Autodesk Inventor part; units mm, degrees
ref_plane "Work Plane1" through (0, 25, 0) normal (0, 1, 0) x (-1, 0, 0)
ref_plane "YZ Plane" through (0, 0, 0) normal (1, 0, 0) x (0, 1, 0)
ref_plane "XY Plane" through (0, 0, 0) normal (0, 0, 1) x (1, 0, 0)
sketch "Sketch1" plane through (0, 0, 0) normal (0, 1, 0) x (-1, 0, 0)
  line L0 (20, 50) -> (-20, 50)
  line L1 (-20, 50) -> (-20, -50)
  line L2 (-20, -50) -> (20, -50)
  line L3 (20, -50) -> (20, 50)
  line L4 (15, 45) -> (-15, 45)
  line L5 (-15, 45) -> (-15, -45)
  line L6 (-15, -45) -> (15, -45)
  line L7 (15, -45) -> (15, 45)
  line L8 (15, -45) -> (15, -50)
  line L9 (-15, -45) -> (-15, -50)
  point P0 (0, 0)
  dimension "d0" = 40
  dimension "d1" = 100
  dimension "d2" = 20
  dimension "d3" = 50
  dimension "d4" = 5
extrude "Extrusion1" add sketch "Sketch1" along normal blind 50 contours L3 L2 L8 L7 L4 L5 L9 L1 L0
sketch "Sketch2" plane through (-20, 0, 50) normal (0, 0, 1) x (1, 0, 0)
  circle A0 centre (20, 33) radius 4
  circle A1 centre (20, 17) radius 4
  circle A2 centre (32, 25) radius 1
  line L0 (0, 0) -> (40, 0)
  line L1 (40, 0) -> (40, 50)
  point P0 (20, 0)
  point P1 (20, 0)
  point P2 (20, 0)
  dimension "d7" = 8
  dimension "d8" = 8
  dimension "d9" = 2
  dimension "d10" = 0
  dimension "d11" = 0
  dimension "d12" = 8
  dimension "d13" = 25
  dimension "d14" = 16
  dimension "d15" = 8
extrude "Extrusion2" cut sketch "Sketch2" against normal up to surface (5 mm away)
sketch "Sketch3" plane through (-20, 0, 50) normal (0, 0, 1) x (1, 0, 0)
  circle A0 centre (20, 33) radius 4
  circle A1 centre (20, 33) radius 6
  circle A2 centre (20, 17) radius 4
  circle A3 centre (20, 17) radius 6
  point P0 (20, 0)
  dimension "d18" = 12
  dimension "d19" = 12
extrude "Extrusion3" add sketch "Sketch3" against normal blind 8
sketch "Sketch4" plane through (-15, 0, -50) normal (0, 0, -1) x (-1, 0, 0)
  circle A0 centre (2.5, 47.5) radius 1.5
  line L0 (5, 0) -> (5, 50)
  line L1 (0, 50) -> (5, 50)
  circle A1 centre (-32.5, 47.5) radius 1.5
  line L2 (-35, 50) -> (-30, 50)
  line L3 (-35, 0) -> (-35, 50)
  circle A2 centre (-32.5, 2.5) radius 1.5
  circle A3 centre (2.5, 2.5) radius 1.5
  line L4 (-35, 0) -> (-30, 0)
  line L5 (0, 0) -> (5, 0)
  point P0 (-15, 0)
  point P1 (-32.5, 50)
  dimension "d22" = 3
  dimension "d23" = 2.5
  dimension "d24" = 2.5
  dimension "d25" = 3
  dimension "d26" = 2.5
  dimension "d27" = 2.5
  dimension "d28" = 3
  dimension "d29" = 3
  dimension "d30" = 2.5
  dimension "d31" = 2.5
  dimension "d32" = 2.5
  dimension "d33" = 2.5
extrude "Extrusion4" cut sketch "Sketch4" against normal blind 5
sketch "Sketch5" plane through (-20, 0, -50) normal (-1, 0, 0) x (0, 0, 1)
  circle A0 centre (15, 33) radius 1.1
  circle A1 centre (70.5, 33) radius 1.1
  circle A2 centre (15, 17) radius 1.1
  circle A3 centre (70.5, 17) radius 1.1
  line L0 (0, 0) -> (0, 50)
  line L1 (0, 0) -> (100, 0)
  point P0 (50, 0)
  dimension "d36" = 2.2
  dimension "d37" = 2.2
  dimension "d38" = 2.2
  dimension "d39" = 2.2
  dimension "d40" = 55.5
  dimension "d41" = 0
  dimension "d42" = 55.5
  dimension "d43" = 16
  dimension "d44" = 16
  dimension "d45" = 0
  dimension "d46" = 15
  dimension "d47" = 17
extrude "Extrusion5" cut sketch "Sketch5" against normal through all
sketch "Sketch6" plane through (0, 50, 0) normal (0, 1, 0) x (1, 0, 0)
  circle A0 centre (10, -47.5) radius 1.5
  circle A1 centre (-10, -47.5) radius 1.5
  line L0 (-20, -50) -> (20, -50)
  circle A2 centre (17.5, 2.5) radius 1.5
  line L1 (20, -50) -> (20, 50)
  circle A3 centre (-17.5, 2.5) radius 1.5
  line L2 (-20, 50) -> (-20, -50)
  line L3 (20, 50) -> (15, 50)
  line L4 (-15, 50) -> (-20, 50)
  point P0 (0, 0)
  point P1 (0, -50)
  point P2 (0, -50)
  dimension "d50" = 3
  dimension "d51" = 3
  dimension "d52" = 2.5
  dimension "d53" = 2.5
  dimension "d54" = 10
  dimension "d55" = 10
  dimension "d56" = 3
  dimension "d57" = 2.5
  dimension "d58" = 3
  dimension "d59" = 2.5
  dimension "d60" = 47.5
  dimension "d61" = 47.5
extrude "Extrusion6" cut sketch "Sketch6" against normal blind 5
ref_plane "Work Plane1" through (0, 25, 0) normal (0, 1, 0) x (-1, 0, 0)
mirror "Mirror1" about plane through (0, 25, 0) normal (0, 1, 0) of "Extrusion6"
properties part number "Handle_Main_Body" material "ABS Plastic"
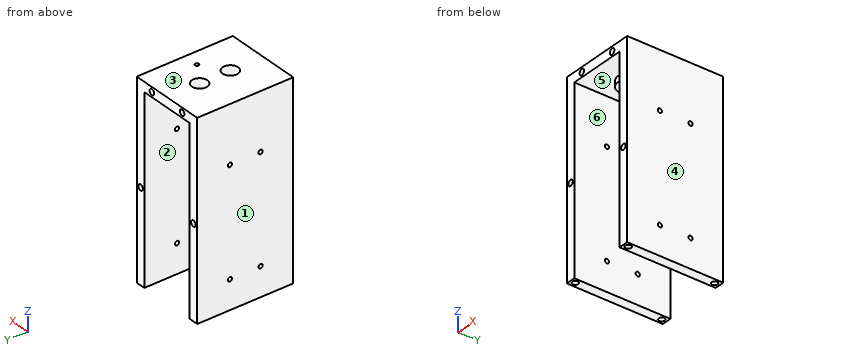
Build history of the part. All positions in model axes, mm. Face numbers are marked on the shaded views. A direction names the side the tool comes from. Round coordinates to 2 decimals unless told otherwise and drop trailing zeros. Write each loop counter-clockwise with the first axis right and the second up, starting at its lowest first coordinate (ties: lowest second). Pieces come first, ordered by that corner, then holes. Notation, with made-up numbers: (-22, -4) -> (21, -4) arc R19 cw to (21, 27) -> close; hole circle Ø11 at (79.5, 30.25). An arc over 180 degrees is marked (long way). Write item = value, one per line.
(1) Two-plate mould, pull along X, no slides. Class the marked faces 1, 2, 3 and 4: pulls with the +X half, pulls with the -X half, needs draft (parallel to the pull), parting line crosses it, or undercut.
Answer:
face_1 = pulls with the -X half
face_2 = undercut
face_3 = needs draft
face_4 = pulls with the +X half
(2) Band-saw the part on D-D (z = 33). Give the cut face in (x, y).
Answer:
outline = (-20, 0) -> (-15, 0) -> (-15, 50) -> (-20, 50) -> close; (15, 0) -> (20, 0) -> (20, 50) -> (15, 50) -> close
(3) Probe L1, parallel to X at y = 5.5, z = 26.5; L2, parallel to Y at x = 16, z = 20; L3, parallel to X at y = 16, z = 43. List the from-to ranges inside material, lowest first.
Answer:
L1 = -20 to -15, 15 to 20
L2 = 0 to 16.02, 17.98 to 32.02, 33.98 to 50
L3 = -20 to -15, -5.92 to -3.87, 3.87 to 5.92, 15 to 20
(4) Band-saw the part on B-B (x = -17.5). Give the cut face in (y, z).
Answer:
outline = (0, -50) -> (1, -50) -> (1, -45) -> (4, -45) -> (4, -50) -> (46, -50) -> (46, -45) -> (49, -45) -> (49, -50) -> (50, -50) -> (50, -4) -> (45, -4) -> (45, -1) -> (50, -1) -> (50, 50) -> (0, 50) -> (0, -1) -> (5, -1) -> (5, -4) -> (0, -4) -> close; hole circle Ø2.2 at (17, -35); hole circle Ø2.2 at (17, 20.5); hole circle Ø2.2 at (33, -35); hole circle Ø2.2 at (33, 20.5)
(5) Band-saw the part on C-C (y = 25). Give the cut face in (x, z).
Answer:
outline = (-20, -50) -> (-15, -50) -> (-15, 45) -> (11, 45) -> (11, 50) -> (-20, 50) -> close; (13, 45) -> (15, 45) -> (15, -50) -> (20, -50) -> (20, 50) -> (13, 50) -> close
(6) Band-saw the part on A-A (z = -35). Give the cut face in (x, y), then the cut area to 3 significant figures.
Answer:
outline = (-20, 0) -> (-15, 0) -> (-15, 15.9) -> (-20, 15.9) -> close; (-20, 18.1) -> (-15, 18.1) -> (-15, 31.9) -> (-20, 31.9) -> close; (-20, 34.1) -> (-15, 34.1) -> (-15, 50) -> (-20, 50) -> close; (15, 0) -> (20, 0) -> (20, 15.9) -> (15, 15.9) -> close; (15, 18.1) -> (20, 18.1) -> (20, 31.9) -> (15, 31.9) -> close; (15, 34.1) -> (20, 34.1) -> (20, 50) -> (15, 50) -> close
area = 456 mm2
(7) Flat gauge pins, fed straight in: pin 1 (2.5 mm diameter, centred on x = -10, z = 47.5, fed in from +Y); pin 2 (9 mm diameter, centred on x = 4.5, y = 19, fed in from -Z); pin 3 (2.5 mm diameter, centred on x = 17.5, y = 47.5, fed in from -Z). Where does each tip first touch, or does it go through?
Answer:
pin_1 = 45
pin_2 = 42
pin_3 = -45
(8) Tool access for the marked faces 5 and 6: list every direction of +Z, -Z, +X, -X, +Y, -Y with a clear straight run to the whole face (end or side of a thin tool).
Answer:
face_5 = -Z
face_6 = -Z, +Y, -Y
